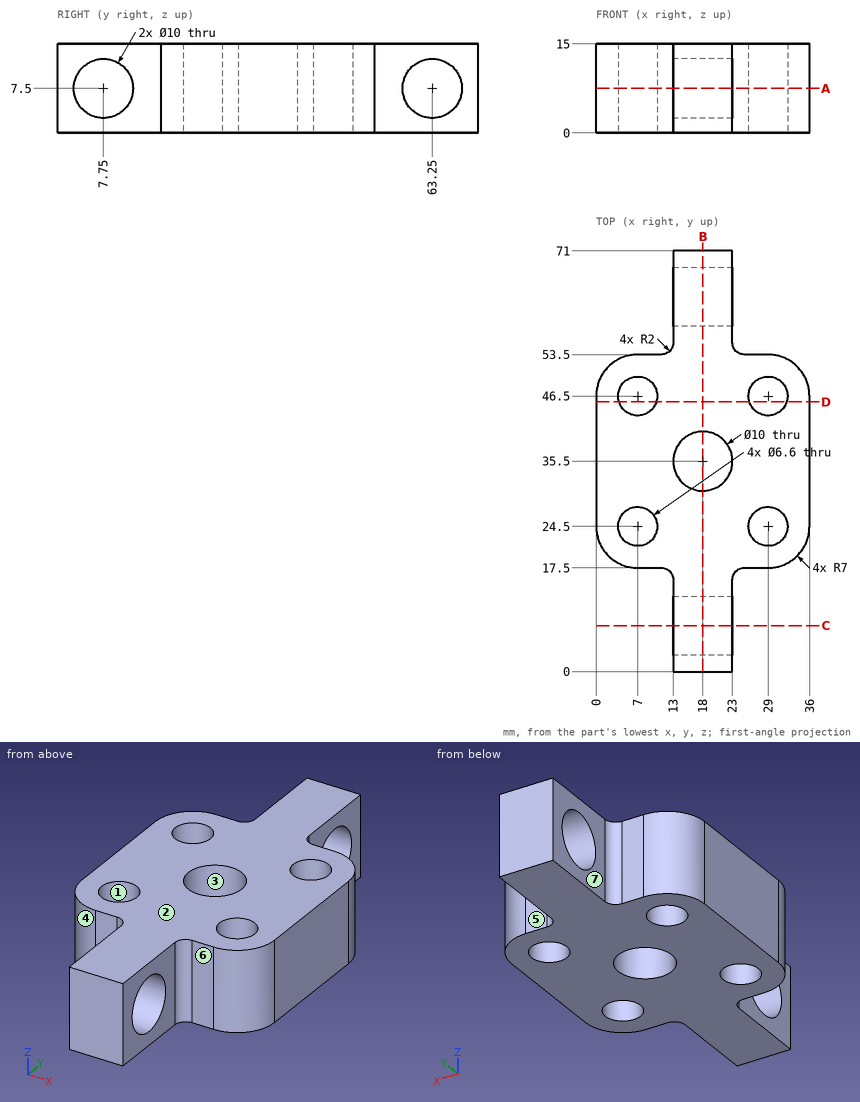
Answer from the drawing. Dimensions are ordinates in mm from the lowest x, y and z of the part. A direction names the side the tool comes from. Round coordinates to 2 decimals unless told otherwise and drop trailing zeros. Loops run counter-clockwise (first coordinate to the right, second up) from the corner with the lowest first, then second, coordinate; pieces in that order, holes last.
1) A cutting plane is placed at A-A on z = 7.5. Give the number of separate pieces and of enclosed holes in the cut face, plus the area to 3 significant figures.
Outcome:
separate pieces: 3
enclosed holes: 5
area: 1,190 mm2
2) Given P1, Ø2, axis at x = 27.5, z = 11, coming from the +Y side; P2, Ø2, axis at x = 10.5, z = 2, coming from the +Y side; P3, Ø3, axis at x = 9.5, z = 8, coming from the -Y side, each flat-ended and moving along its own axis, determine where each tip first touches the part or whether it passes through.
Outcome:
P1: stops at y = 53.5
P2: stops at y = 53.56
P3: stops at y = 17.5
3) A cutting plane is placed at C-C on y = 7.75. Determine the outline of the cut face in (x, z).
Outcome:
outline: (13, 0) - (23, 0) - (23, 2.5) - (13, 2.5) - close; (13, 12.5) - (23, 12.5) - (23, 15) - (13, 15) - close
4) A cutting plane is placed at B-B on x = 18. Determine the outline of the cut face in (y, z).
Outcome:
outline: (0, 0) - (30.5, 0) - (30.5, 15) - (0, 15) - close; (40.5, 0) - (71, 0) - (71, 15) - (40.5, 15) - close; hole circle Ø10 at (7.75, 7.5); hole circle Ø10 at (63.25, 7.5)
5) For a pull along Y with two mould halves and no side action, classify the marked faces 1, 2, 3 and 4 as released by +Y, released by -Y, zero draft, split by the parting line, or undercut.
Outcome:
face 1: undercut
face 2: zero draft
face 3: undercut
face 4: released by -Y
6) For the marked faces 5, 6 and 7, determine the directions among +Z, -Z, +X, -X, +Y, -Y from which every point of the face is accessible in a straight line to the end or side of a thin tool.
Outcome:
face 5: +Z, -Z, +X, +Y
face 6: +Z, -Z, +X, -Y
face 7: +Z, -Z, -X, +Y
7) A cutting plane is placed at D-D on y = 45.5. Determine the outline of the cut face in (x, z), plus the area to 3 significant figures.
Outcome:
outline: (0, 0) - (3.86, 0) - (3.86, 15) - (0, 15) - close; (10.14, 0) - (25.86, 0) - (25.86, 15) - (10.14, 15) - close; (32.14, 0) - (36, 0) - (36, 15) - (32.14, 15) - close
area: 351 mm2
8) Consider line 1 (Y direction, x = 7, z = 7.25); line 2 (Y direction, x = 16.5, z = 10.5); line 3 (Y direction, x = 18.5, z = 8). Determine where each line is inside the solid, lowest interval first.
Outcome:
line 1: y = 17.5 to 21.2, 27.8 to 43.2, 49.8 to 53.5
line 2: y = 0 to 3.75, 11.75 to 30.73, 40.27 to 59.25, 67.25 to 71
line 3: y = 0 to 2.78, 12.72 to 30.53, 40.47 to 58.28, 68.22 to 71
